The model under review builds one solid part; all positions refer to its coordinate system, in mm. A direction names the side the tool comes from. Give positions to 0.01 mm unless a question says otherwise; leave off trailing zeros. Write each loop counter-clockwise with the first axis right and the second up, starting at its lowest first coordinate (ties: lowest second). Pieces come first, ordered by that corner, then holes. Notation, with made-up numbers: (56.5, 65) - (87.5, 65) arc R8 ccw to (87.5, 77) - close; hole circle Ø8 at (53.25, 76.25). An arc over 180 degrees is marked (long way). Write item = value, one per line.
```python
from build123d import *

# Parameters (mm, degrees)
RESSALTO_EXTRUS_O1_DEPTH = 1
RESSALTO_EXTRUS_O3_DEPTH = 6


with BuildPart() as part:
    # Esboço1 → Ressalto-extrusão1 (new body)
    with BuildSketch(Plane.XY):
        with BuildLine():
            Line((0, 1.869246597), (-27.993590125, 22.6849931))
            Line((-27.993590125, 22.6849931), (-28.177477369, 22.821729769))
            ThreePointArc((-28.177477369, 22.821729769), (-29.024277982, 26.673027959), (-32.763028277, 27.926549102))
            ThreePointArc((-32.763028277, 27.926549102), (-39.996629104, 28.442571725), (-35.736971723, 22.573450898))
            ThreePointArc((-35.736971723, 22.573450898), (-33.37897048, 20.245211003), (-30.074575689, 20.493899428))
            Line((-30.074575689, 20.493899428), (-29.783698424, 20.277606077))
            Line((-29.783698424, 20.277606077), (-2.513814389, 0))
            Line((-2.513814389, 0), (-29.783698424, -20.277606077))
            Line((-29.783698424, -20.277606077), (-30.074575689, -20.493899428))
            ThreePointArc((-30.074575689, -20.493899428), (-33.37897048, -20.245211003), (-35.736971723, -22.573450898))
            ThreePointArc((-35.736971723, -22.573450898), (-39.996629104, -28.442571725), (-32.763028277, -27.926549102))
            ThreePointArc((-32.763028277, -27.926549102), (-29.024277982, -26.673027959), (-28.177477369, -22.821729769))
            Line((-28.177477369, -22.821729769), (-27.993590125, -22.6849931))
            Line((-27.993590125, -22.6849931), (0, -1.869246597))
            Line((0, -1.869246597), (1, -1.869246597))
            Line((1, -1.869246597), (28.993590125, -22.6849931))
            Line((28.993590125, -22.6849931), (29.177477369, -22.821729769))
            ThreePointArc((29.177477369, -22.821729769), (30.024277982, -26.673027959), (33.763028277, -27.926549102))
            ThreePointArc((33.763028277, -27.926549102), (40.996629104, -28.442571725), (36.736971723, -22.573450898))
            ThreePointArc((36.736971723, -22.573450898), (34.37897048, -20.245211003), (31.074575689, -20.493899428))
            Line((31.074575689, -20.493899428), (30.783698424, -20.277606077))
            Line((30.783698424, -20.277606077), (3.513814389, 0))
            Line((3.513814389, 0), (30.783698424, 20.277606077))
            Line((30.783698424, 20.277606077), (31.074575689, 20.493899428))
            ThreePointArc((31.074575689, 20.493899428), (34.37897048, 20.245211003), (36.736971723, 22.573450898))
            ThreePointArc((36.736971723, 22.573450898), (40.996629104, 28.442571725), (33.763028277, 27.926549102))
            ThreePointArc((33.763028277, 27.926549102), (30.024277982, 26.673027959), (29.177477369, 22.821729769))
            Line((29.177477369, 22.821729769), (28.993590125, 22.6849931))
            Line((28.993590125, 22.6849931), (1, 1.869246597))
            Line((1, 1.869246597), (0, 1.869246597))
        make_face()
        Polygon((-38.479898987, 26.5), (-36.5, 28.479898987), (-34.520101013, 26.5), (-36.5, 24.520101013), align=None, mode=Mode.SUBTRACT)
        Polygon((-33.979898987, 24), (-32, 25.979898987), (-30.020101013, 24), (-32, 22.020101013), align=None, mode=Mode.SUBTRACT)
        Polygon((-36.5, -28.479898987), (-34.520101013, -26.5), (-36.5, -24.520101013), (-38.479898987, -26.5), align=None, mode=Mode.SUBTRACT)
        Polygon((-32, -25.979898987), (-30.020101013, -24), (-32, -22.020101013), (-33.979898987, -24), align=None, mode=Mode.SUBTRACT)
        Polygon((39.479898987, -26.5), (37.5, -28.479898987), (35.520101013, -26.5), (37.5, -24.520101013), align=None, mode=Mode.SUBTRACT)
        Polygon((34.979898987, -24), (33, -25.979898987), (31.020101013, -24), (33, -22.020101013), align=None, mode=Mode.SUBTRACT)
        Polygon((37.5, 28.479898987), (35.520101013, 26.5), (37.5, 24.520101013), (39.479898987, 26.5), align=None, mode=Mode.SUBTRACT)
        Polygon((33, 25.979898987), (31.020101013, 24), (33, 22.020101013), (34.979898987, 24), align=None, mode=Mode.SUBTRACT)
    extrude(amount=RESSALTO_EXTRUS_O1_DEPTH)

    # Esboço3 → Ressalto-extrusão3 (add)
    # profile 1 of 4: a face of its own
    with BuildSketch(Plane.XY.offset(1)):
        with BuildLine():
            ThreePointArc((-32.525798154, 26.953563323), (-39.996629104, 28.442571725), (-34.785522601, 22.886059319))
            ThreePointArc((-34.785522601, 22.886059319), (-34.622471828, 25.456928794), (-32.525798154, 26.953563323))
        make_face()
        Polygon((-38.479898987, 26.5), (-36.5, 24.520101013), (-34.520101013, 26.5), (-36.5, 28.479898987), align=None, mode=Mode.SUBTRACT)
    # profile 2 of 4: a face of its own
    with BuildSketch(Plane.XY.offset(1)):
        with BuildLine():
            ThreePointArc((-32.525798154, -26.953563323), (-34.622471828, -25.456928794), (-34.785522601, -22.886059319))
            ThreePointArc((-34.785522601, -22.886059319), (-39.996629104, -28.442571725), (-32.525798154, -26.953563323))
        make_face()
        Polygon((-36.5, -24.520101013), (-34.520101013, -26.5), (-36.5, -28.479898987), (-38.479898987, -26.5), align=None, mode=Mode.SUBTRACT)
    # profile 3 of 4: a face of its own
    with BuildSketch(Plane.XY.offset(1)):
        with BuildLine():
            ThreePointArc((33.525798154, -26.953563323), (40.996629104, -28.442571725), (35.785522601, -22.886059319))
            ThreePointArc((35.785522601, -22.886059319), (35.622471828, -25.456928794), (33.525798154, -26.953563323))
        make_face()
        Polygon((39.479898987, -26.5), (37.5, -24.520101013), (35.520101013, -26.5), (37.5, -28.479898987), align=None, mode=Mode.SUBTRACT)
    # profile 4 of 4: a face of its own
    with BuildSketch(Plane.XY.offset(1)):
        with BuildLine():
            ThreePointArc((33.525798154, 26.953563323), (35.622471828, 25.456928794), (35.785522601, 22.886059319))
            ThreePointArc((35.785522601, 22.886059319), (40.996629104, 28.442571725), (33.525798154, 26.953563323))
        make_face()
        Polygon((37.5, 24.520101013), (35.520101013, 26.5), (37.5, 28.479898987), (39.479898987, 26.5), align=None, mode=Mode.SUBTRACT)
    extrude(amount=RESSALTO_EXTRUS_O3_DEPTH)


solid = part.part
```
1. Machinability: for faces 4 (the flat face through (-35.52, -27.5, 3.45)), 5 (the cylindrical face through (-34.6, -25.5, 4)), which of the approach directions +Z, -Z, +X, -X, +Y, -Y give a long, thin tool a straight path to every point of the face, cutting with its end or side? Answer none if there is none.
Findings below:
face_4 = +Z, -Z
face_5 = +Z
2. For line 1 (Y direction, x = 37, z = 1.75); line 2 (Y direction, x = 38.5, z = 2.25); line 3 (Y direction, x = -34, z = 4), list the stretches that pass through material, from the lowest coordinate up. Write a range as from..to.
Findings below:
line_1 = -30.47..-27.98, -25.02..-22.53, 22.53..25.02, 27.98..30.47
line_2 = -30.37..-27.48, -25.52..-22.63, 22.63..25.52, 27.48..30.37
line_3 = -29.62..-26.24, 26.24..29.62
3. Insertion check: P1, Ø1.1, axis at x = 0.5, z = 0.5, coming from the -Y side; P2, Ø3, axis at x = -21.5, z = 2, coming from the +Y side; P3, Ø1.1, axis at x = 0.5, z = 0.5, coming from the +Y side; P4, Ø4, axis at x = 4, y = 9, coming from the -Z side. Each pin has a flat end and moves straight along its axis. Give the tip position at first contact, or say it passes through.
Findings below:
P1 = -1.91
P2 = 18.69
P3 = 1.91
P4 = through
4. Draft analysis for pull direction Y (two halves, no side actions). For faces 1 (the cylindrical face through (35.6, 25.5, 4)), 2 (the flat face through (38.48, -25.5, 3.45)), 3 (the flat face through (-38.3, 27.4, 7)), state which applies: +Y half, -Y half, draft (parallel to the pull), parting line (faces both ways), or undercut.
Findings below:
face_1 = undercut
face_2 = undercut
face_3 = draft
5. Take a section at B-B on y = 5.5. Give the boundary of the cut face in (x, z), and give its area (3 significant figures).
Findings below:
outline = (-9.91, 0) - (-4.88, 0) - (-4.88, 1) - (-9.91, 1) - close; (5.88, 0) - (10.91, 0) - (10.91, 1) - (5.88, 1) - close
area = 10.1 mm²
6. Take a section at C-C on x = 21.5. Give the boundary of the cut face in (y, z).
Findings below:
outline = (-17.11, 0) - (-13.37, 0) - (-13.37, 1) - (-17.11, 1) - close; (13.37, 0) - (17.11, 0) - (17.11, 1) - (13.37, 1) - close
7. Take a section at A-A on z = 4.75. Give the boundary of the cut face in (x, y).
Findings below:
outline = (-34.79, -22.89) arc R4 ccw (long way) to (-32.53, -26.95) arc R3 cw to start; (-34.79, 22.89) arc R3 cw to (-32.53, 26.95) arc R4 ccw (long way) to start; (33.53, -26.95) arc R4 ccw (long way) to (35.79, -22.89) arc R3 cw to start; (33.53, 26.95) arc R3 cw to (35.79, 22.89) arc R4 ccw (long way) to start; hole (-38.48, -26.5) - (-36.5, -28.48) - (-34.52, -26.5) - (-36.5, -24.52) - close; hole (-38.48, 26.5) - (-36.5, 24.52) - (-34.52, 26.5) - (-36.5, 28.48) - close; hole (35.52, -26.5) - (37.5, -28.48) - (39.48, -26.5) - (37.5, -24.52) - close; hole (35.52, 26.5) - (37.5, 24.52) - (39.48, 26.5) - (37.5, 28.48) - close
